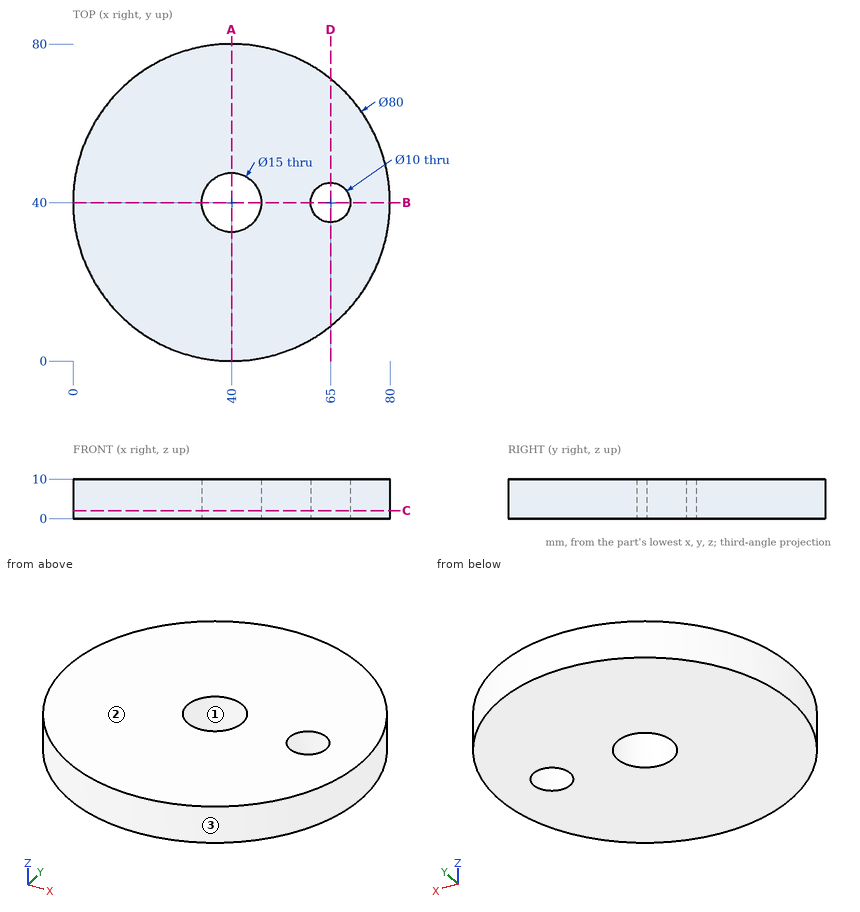
Check sheet for the drawn part. Datum: minimum x, y, z corner. Units: mm. Give positions to 0.01 mm unless a question says otherwise; leave off trailing zeros. Write each loop counter-clockwise with the first axis right and the second up, starting at its lowest first coordinate (ties: lowest second). Pieces come first, ordered by that corner, then holes. Notation, with made-up numbers: M 68,-2 L 125,-2 A8 cw 125,7 Z; hole C -30,45.25 d7. An arc over 180 degrees is marked long. One line per question, with ' | ' between items.
1. Cross-section at B-B (y = 40). Enter the section's corners in (x, z), plus the area to 3 significant figures.
Ans:
outline: M 0,0 L 32.5,0 L 32.5,10 L 0,10 Z; M 47.5,0 L 60,0 L 60,10 L 47.5,10 Z; M 70,0 L 80,0 L 80,10 L 70,10 Z | area: 550 mm2
2. Cross-section at D-D (x = 65). Enter the section's corners in (y, z).
Ans:
outline: M 8.78,0 L 35,0 L 35,10 L 8.78,10 Z; M 45,0 L 71.22,0 L 71.22,10 L 45,10 Z
3. Scan lines: line 1 along X through (y, z) = (41, 9.25); line 2 along X through (y, z) = (38.5, 8.75); line 3 along Y through (x, z) = (40, 4.5). Record each from-to range of solid material in increasing order. Write a range as from..to.
Ans:
line 1: 0.01..32.57, 47.43..60.1, 69.9..79.99 | line 2: 0.03..32.65, 47.35..60.23, 69.77..79.97 | line 3: 0..32.5, 47.5..80
4. Gauge pin test, flat ends, axial feed: pin 1 (4 mm diameter, centred on x = 40, z = 1.5, fed in from +Y); pin 2 (4 mm diameter, centred on x = 13.5, z = 2.5, fed in from +Y); pin 3 (1 mm diameter, centred on x = 71.5, z = 2.5, fed in from +Y). Record the tip position at first contact, or that the pin passes through.
Ans:
pin 1: y = 80 | pin 2: y = 71.62 | pin 3: y = 65.28
5. Mould release check, pull along X, two halves, no side actions. Record for the marked faces 1, 2 and 3: released by +X, released by -X, zero draft, split by the parting line, or undercut.
Ans:
face 1: undercut | face 2: zero draft | face 3: split by the parting line
6. Cross-section at A-A (x = 40). Enter the section's corners in (y, z).
Ans:
outline: M 0,0 L 32.5,0 L 32.5,10 L 0,10 Z; M 47.5,0 L 80,0 L 80,10 L 47.5,10 Z
7. Cross-section at C-C (z = 2). Enter the section's corners in (x, y).
Ans:
outline: C 40,40 d80; hole C 40,40 d15; hole C 65,40 d10
